```python
from build123d import *

# Parameters (mm, degrees)
ESQUISSE1_W        = 20
ESQUISSE1_H        = 20
BOSS_EXTRU_1_DEPTH = 9
BOSS_EXTRU_2_DEPTH = 1
CHANFREIN1_SIZE    = 0.2
ESQUISSE4_R        = 1.8000000000000007
BOSS_EXTRU_3_DEPTH = 6


with BuildPart() as part:
    # Esquisse1 → Boss.-Extru.1 (new body)
    with BuildSketch(Plane.XY):
        with Locations((10, 10)):
            Rectangle(ESQUISSE1_W, ESQUISSE1_H)
    extrude(amount=BOSS_EXTRU_1_DEPTH)

    # Esquisse2 → Boss.-Extru.2 (add)
    with BuildSketch(Plane(origin=(0, 20, 0), x_dir=(1, 0, 0), z_dir=(0, 1, 0))):
        with BuildLine():
            ThreePointArc((7.256081239041076, -2.4695268848630905), (5.0000000000000115, -1.4647531190285523), (2.7439187609589397, -2.469526884863073))
            Line((2.743918760958954, -2.4695268848630585), (5.000000000000001, -4.500000000000001))
            Line((5.000000000000001, -4.499999999999999), (7.256081239041048, -2.4695268848630567))
        make_face()
        with BuildLine():
            Line((5.000000000000001, -4.500000000000001), (2.743918760958954, -2.4695268848630585))
            ThreePointArc((2.7439187609589397, -2.469526884863073), (1.9647531190285523, -4.5), (2.743918760958939, -6.530473115136926))
            Line((2.743918760958954, -6.5304731151369415), (5.000000000000001, -4.499999999999999))
        make_face()
        with BuildLine():
            Line((7.256081239041048, -2.4695268848630567), (5.000000000000001, -4.499999999999999))
            Line((5.000000000000001, -4.500000000000001), (7.256081239041048, -6.530473115136943))
            ThreePointArc((7.256081239041075, -6.53047311513691), (7.833768442592348, -5.587418981908373), (8.035246880971448, -4.500000000000001))
            ThreePointArc((8.035246880971448, -4.5), (7.833768442592348, -3.412581018091629), (7.256081239041075, -2.46952688486309))
        make_face()
        with BuildLine():
            Line((7.256081239041048, -6.530473115136943), (5.000000000000001, -4.500000000000001))
            Line((5.000000000000001, -4.499999999999999), (2.743918760958954, -6.5304731151369415))
            ThreePointArc((2.743918760958939, -6.530473115136926), (5.000000000000011, -7.535246880971448), (7.256081239041075, -6.53047311513691))
        make_face()
    extrude(amount=BOSS_EXTRU_2_DEPTH)

    # Chanfrein1
    chanfrein1_edges = [part.edges().sort_by_distance(p)[0] for p in [
        (7.256081239041057, 21, 2.469526884863065),
    ]]
    chamfer(chanfrein1_edges, length=CHANFREIN1_SIZE)

    # Esquisse4 → Boss.-Extru.3 (add)
    with BuildSketch(Plane(origin=(0, 21, 0), x_dir=(1, 0, 0), z_dir=(0, 1, 0))):
        with Locations(Location((5, -4.5, 0), (0, 0, 270))):
            Circle(ESQUISSE4_R)
    extrude(amount=BOSS_EXTRU_3_DEPTH)


solid = part.part
```
Geometry: final body of the model. Coordinates: model frame, mm. A direction names the side the tool comes from. Give positions to 0.01 mm unless a question says otherwise; leave off trailing zeros. Loops run counter-clockwise (first coordinate to the right, second up) from the corner with the lowest first, then second, coordinate; pieces in that order, holes last. Notation, with made-up numbers: (25, -12) -> (62, -12) arc R31 cw to (62, 20) -> close; hole circle Ø4 at (-34.75, -26). An arc over 180 degrees is marked (long way). Use CSV: the item, a comma, the result in double quotes.
(1) Cut plane C-C (y = 24.5). Output: boundary loops of the cut face in (x, z), plus the area to 3 significant figures.
From the geometry:
outline,"circle Ø3.6 at (5, 4.5)"
area,"10.2 mm^2"
(2) Access query for faces 1 (the face through (10, 10, 9)), 2 (the face through (2.24, 20.39, 3.24)). Directions: +Z, -Z, +X, -X, +Y, -Y. A direction counts if a zero-diameter tool reaches every point of the face in a straight line with its end or side. Return the directions, or none.
From the geometry:
face 1,"+Z, +X, -X, +Y, -Y"
face 2,"+Y"
(3) Ray query, line 1 along Y through (x, z) = (3.5, 6); line 2 along Y through (x, z) = (8.5, 5.25); line 3 along X through (y, z) = (20.75, 4.5). Return the intervals inside material, ascending. Write a range as [from, to].
From the geometry:
line 1,"[0, 21]"
line 2,"[0, 20]"
line 3,"[1.96, 8.04]"
(4) Cut plane A-A (z = 4.5). Output: boundary loops of the cut face in (x, y).
From the geometry:
outline,"(0, 0) -> (20, 0) -> (20, 20) -> (8.04, 20) -> (8.04, 20.8) -> (7.84, 21) -> (6.8, 21) -> (6.8, 27) -> (3.2, 27) -> (3.2, 21) -> (2.16, 21) -> (1.96, 20.8) -> (1.96, 20) -> (0, 20) -> close"
(5) Cut plane B-B (x = 5). Output: boundary loops of the cut face in (y, z).
From the geometry:
outline,"(0, 0) -> (20, 0) -> (20, 1.46) -> (20.8, 1.46) -> (21, 1.66) -> (21, 2.7) -> (27, 2.7) -> (27, 6.3) -> (21, 6.3) -> (21, 7.34) -> (20.8, 7.54) -> (20, 7.54) -> (20, 9) -> (0, 9) -> close"
(6) Cut plane D-D (x = 10). Output: boundary loops of the cut face in (y, z), plus the area to 3 significant figures.
From the geometry:
outline,"(0, 0) -> (20, 0) -> (20, 9) -> (0, 9) -> close"
area,"180 mm^2"
